Work out the finished part from the listing and answer in its coordinate system (mm). Face numbers are marked on the shaded views. Give positions to 0.01 mm unless a question says otherwise; leave off trailing zeros. Order: outer loops, then holes, each group sorted by start corner. A loop starts at its lowest first (then second) coordinate and runs counter-clockwise, first axis right, second up. Notation, with made-up numbers: M 39.5,64.25 L 78.5,64.25 A11 ccw 78.5,75.25 Z; hole C 6.25,70 d1. An arc over 180 degrees is marked long. One line per item, written item: value.
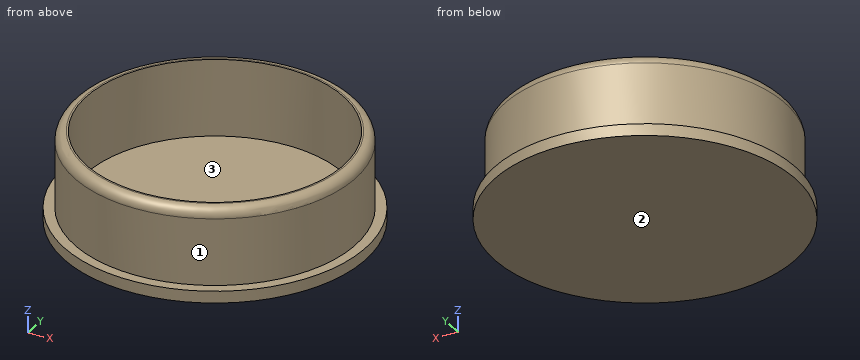
from build123d import *

# Parameters (mm, degrees)
F0_R     = 25.5
F0_R_2   = 23.75
F0_R_3   = 21.75
F1_DEPTH = 2
F2_DEPTH = 15
F3_R     = 1.7


with BuildPart() as f1:
    # F0 (on Top) → F1 (new body)
    with BuildSketch(Plane.XY):
        Circle(F0_R)
        Circle(F0_R_2, mode=Mode.SUBTRACT)
        Circle(F0_R_2)
        Circle(F0_R_3, mode=Mode.SUBTRACT)
        Circle(F0_R_3)
    extrude(amount=F1_DEPTH)

    # F0 (on Top) → F2 (join)
    with BuildSketch(Plane.XY):
        Circle(F0_R_2)
        Circle(F0_R_3, mode=Mode.SUBTRACT)
    extrude(amount=F2_DEPTH)

    # F3
    f3_edges = [f1.edges().sort_by_distance(p)[0] for p in [
        (-23.75, 0, 15),
    ]]
    fillet(f3_edges, radius=F3_R)


solid = f1.part
(1) Given P1, Ø1, axis at x = 2, y = 3, coming from the +Z side; P2, Ø2, axis at x = 20, z = 3.5, coming from the +Y side; P3, Ø1, axis at x = 1.5, z = 9.5, coming from the -Y side, each flat-ended and moving along its own axis, determine where each tip first touches the part or whether it passes through.
Findings:
P1: stops at z = 2
P2: stops at y = 14.25
P3: stops at y = -23.73
(2) Section A-A, the plane y = 0 is taken. Give the vertices of the cut face in (x, z).
Findings:
outline: M -25.5,0 L 25.5,0 L 25.5,2 L 23.75,2 L 23.75,13.3 A1.7 ccw 22.05,15 L 21.75,15 L 21.75,2 L -21.75,2 L -21.75,15 L -22.05,15 A1.7 ccw -23.75,13.3 L -23.75,2 L -25.5,2 Z
(3) Section C-C, the plane z = 4.5 is taken. Give the vertices of the cut face in (x, y), then the cut area to 3 significant figures.
Findings:
outline: C 0,0 d47.5; hole C 0,0 d43.5
area: 286 mm^2
(4) Section D-D, the plane z = 1 is taken. Give the vertices of the cut face in (x, y), then the cut area to 3 significant figures.
Findings:
outline: C 0,0 d51
area: 2,040 mm^2
(5) Find the intervals of material crossed by probe 1 along Y at (x, z) = (0, 10); probe 2 along Z at (x, y) = (-13, -8), in increasing order. Write a range as from..to.
Findings:
probe 1: y = -23.75..-21.75, 21.75..23.75
probe 2: z = 0..2
(6) Determine the mould class of the marked faces 1, 2 and 3 for opening direction Y: pulls with the +Y half, pulls with the -Y half, needs draft (parallel to the pull), parting line crosses it, or undercut.
Findings:
face 1: parting line crosses it
face 2: needs draft
face 3: undercut
